Can you work these out from the model? Positions are in its coordinate system, mm. A direction names the side the tool comes from. Give positions to 0.01 mm unless a question says otherwise; leave off trailing zeros. Order: outer loops, then holes, each group sorted by start corner. A loop starts at its lowest first (then second) coordinate and runs counter-clockwise, first axis right, second up. Notation, with made-up numbers: (20.25, 86) - (53.25, 86) arc R24 cw to (53.25, 104) - close; hole circle Ø3 at (24.5, -3.5). An arc over 180 degrees is marked (long way). Answer as CSV lines item,"result".
```python
from build123d import *

# Parameters (mm, degrees)
BASPROSKE_W        = 19
BASPROSKE_H        = 22
TOOTHCUT_DEPTH     = 37.455452267
TEETHCUTS_COUNT    = 20
TEETHCUTS_ANGLE    = 342
SKETCH1_R          = 1.85
CUT_EXTRUDE1_DEPTH = 37.221987796


with BuildPart() as part:
    # BasProSke → Base-Revolve (revolve)
    with BuildSketch(Plane(origin=(0, 0, 0), x_dir=(1, 0, 0), z_dir=(0, 1, 0)), mode=Mode.PRIVATE) as base_revolve_sk:
        with Locations((9.5, 11)):
            Rectangle(BASPROSKE_W, BASPROSKE_H)
    revolve(base_revolve_sk.sketch.rotate(Axis((-10, 0, 0), (1, 0, 0)), 180), axis=Axis((-10, 0, 0), (1, 0, 0)))

    # TooCutSke → ToothCut (cut, through all)
    with BuildSketch(Plane(origin=(0, 0, 0), x_dir=(0, 0, -1), z_dir=(1, 0, 0))):
        with BuildLine():
            ThreePointArc((0.986171591, 17.471189616), (0, 17.499), (-0.986171591, 17.471189616))
            ThreePointArc((-0.986171591, 17.471189616), (-1.626916196, 19.798789858), (-2.932850173, 21.829260982))
            ThreePointArc((-2.932850173, 21.829260982), (0, 22.0254), (2.932850173, 21.829260982))
            ThreePointArc((2.932850173, 21.829260982), (1.626916196, 19.798789858), (0.986171591, 17.471189616))
        make_face()
    toothcut = extrude(amount=TOOTHCUT_DEPTH, mode=Mode.SUBTRACT)

    # TeethCuts: ToothCut ×20 about axis
    teethcuts_axis = Axis((-10, 0, 0), (1, 0, 0))
    for i in range(1, TEETHCUTS_COUNT):
        add(toothcut.rotate(teethcuts_axis, i * TEETHCUTS_ANGLE / (TEETHCUTS_COUNT - 1)), mode=Mode.SUBTRACT)

    # Sketch1 → Cut-Extrude1 (cut, through all)
    with BuildSketch(Plane(origin=(19, 0, 0), x_dir=(0, 0, -1), z_dir=(1, 0, 0))):
        Circle(SKETCH1_R)
    extrude(amount=-CUT_EXTRUDE1_DEPTH, mode=Mode.SUBTRACT)


solid = part.part
```
1) Which directions (+Z, -Z, +X, -X, +Y, -Y) give clear straight access to the entire face, cutting with the end or side of a thin tool? Please do faces 1 (the cylindrical face through (9.37, -15.07, 12.97)), 2 (the cylindrical face through (9.367, 15.037, 12.911)), 3 (the cylindrical face through (9.37, 10.31, 16.93)).
Answer block:
face 1,"+X, -X, -Y"
face 2,"+X, -X, +Y"
face 3,"+X, -X"
2) I want a section at D-D on y = 7.5. Write out the boundary of the cut face in (x, z).
Answer block:
outline,"(0, -18.14) - (19, -18.14) - (19, 18.14) - (0, 18.14) - close"
3) I want a section at A-A on z = 0. Write out the boundary of the cut face in (x, y).
Answer block:
outline,"(0, -17.5) - (19, -17.5) - (19, -1.85) - (0, -1.85) - close; (0, 1.85) - (19, 1.85) - (19, 17.5) - (0, 17.5) - close"
4) I'm going to push flat-ended pins straight in: P1, Ø8, axis at x = 11, z = -12.5, coming from the +Y side; P2, Ø6, axis at x = 13, y = -2, coming from the -Z side; P3, Ø3, axis at x = 7, z = -17.5, coming from the -Y side. Where does each tip first touch, or does it pass through?
Answer block:
P1,"y = 19.84"
P2,"z = -21.81"
P3,"y = -10.49"
5) I want a section at C-C on z = -7. Write out the boundary of the cut face in (x, y).
Answer block:
outline,"(0, -17.48) - (19, -17.48) - (19, 17.48) - (0, 17.48) - close"
6) I need wall thicknesses on line 1 along Z through (x, y) = (6.5, 15); line 2 along Z through (x, y) = (6.25, -3); line 3 along Z through (x, y) = (14.75, -7). Which ranges of each line are inside material? Lowest first, please. Write a range as [from, to].
Answer block:
line 1,"[-15.89, -12.85], [-9.62, 9.62], [12.85, 15.89]"
line 2,"[-21.79, 21.79]"
line 3,"[-17.48, 17.48]"
